Drawing for the job (mm, zero at the part's lowest x, y, z). A direction names the side the tool comes from. Coordinates: 2 decimals unless noted, no trailing zeros. Order: outer loops, then holes, each group sorted by start corner. A loop starts at its lowest first (then second) coordinate and runs counter-clockwise, first axis right, second up.
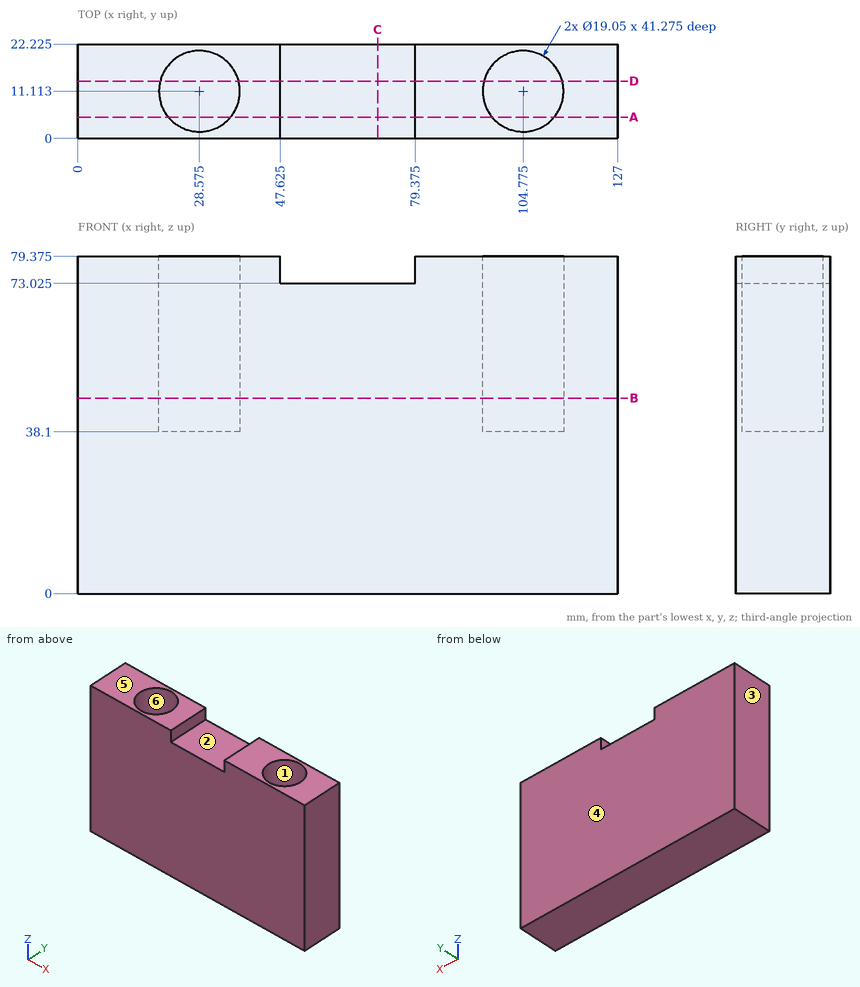
1) Drill centre lines: probe 1 along X at (y, z) = (8.5, 48.5) (1 decimal); probe 2 along X at (y, z) = (18.5, 39) (1 decimal); probe 3 along Z at (x, y) = (51, 11.5) (1 decimal). Where is each one in solid material? Low to high.
2) Pin check, flat tip, straight feed: P1, Ø9.5, axis at x = 24.5, y = 12, coming from the +Z side. Stop position of the tip, or through.
3) Two-plate mould, pull along Y, no slides. Class the marked faces 4, 5 and 6: released by +Y, released by -Y, zero draft, split by the parting line, or undercut.
4) Slice it at D-D (y = 13.5). List the corners of the cut face in (x, z) (1 decimal), plus the area to 3 significant figures.
5) Which spindle directions (+Z, -Z, +X, -X, +Y, -Y) get a long thin tool onto all of the face, cutting with end or side? Do the marked faces 1, 2 and 3. Say none if no direction does.
6) Slice it at B-B (z = 46). Give the number of separate pieces and of enclosed holes in the cut face, plus the area to 3 significant figures.
7) Slice it at A-A (y = 5). List the corners of the cut face in (x, z) (1 decimal).
8) Slice it at C-C (x = 70.5). List the corners of the cut face in (y, z) (1 decimal), plus the area to 3 significant figures.
Worked out:
1. probe 1: x = 0 to 19.4, 37.7 to 95.6, 113.9 to 127
1. probe 2: x = 0 to 22.6, 34.6 to 98.8, 110.8 to 127
1. probe 3: z = 0 to 73
2. P1: stops at z = 38.1
3. face 4: released by +Y
3. face 5: zero draft
3. face 6: undercut
4. outline: (0, 0) - (127, 0) - (127, 79.4) - (114, 79.4) - (114, 38.1) - (95.6, 38.1) - (95.6, 79.4) - (79.4, 79.4) - (79.4, 73) - (47.6, 73) - (47.6, 79.4) - (37.8, 79.4) - (37.8, 38.1) - (19.4, 38.1) - (19.4, 79.4) - (0, 79.4) - close
4. area: 8,360 mm2
5. face 1: +Z
5. face 2: +Z, +Y, -Y
5. face 3: +Z, -Z, -X, +Y, -Y
6. separate pieces: 1
6. enclosed holes: 2
6. area: 2,250 mm2
7. outline: (0, 0) - (127, 0) - (127, 79.4) - (112.1, 79.4) - (112.1, 38.1) - (97.5, 38.1) - (97.5, 79.4) - (79.4, 79.4) - (79.4, 73) - (47.6, 73) - (47.6, 79.4) - (35.9, 79.4) - (35.9, 38.1) - (21.3, 38.1) - (21.3, 79.4) - (0, 79.4) - close
8. outline: (0, 0) - (22.2, 0) - (22.2, 73) - (0, 73) - close
8. area: 1,620 mm2
